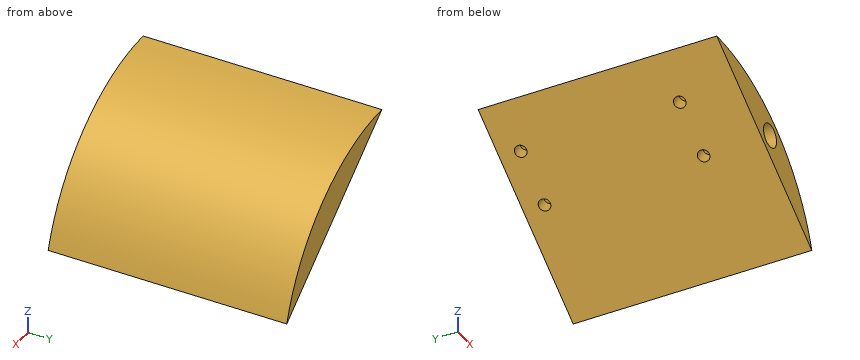
from build123d import *

# Parameters (mm, degrees)
SKETCH1_R           = 85.725
BOSS_EXTRUDE1_DEPTH = 114.3
CUT_EXTRUDE1_DEPTH  = 152.4
SKETCH3_R           = 2.778125
CUT_EXTRUDE2_DEPTH  = 7.9375
SKETCH4_R           = 5.588
CUT_EXTRUDE3_DEPTH  = 6.096


with BuildPart() as part:
    # Sketch1 → Boss-Extrude1 (new body)
    with BuildSketch(Plane(origin=(0, 0, 0), x_dir=(1, 0, 0), z_dir=(0, 1, 0))):
        Circle(SKETCH1_R)
    extrude(amount=BOSS_EXTRUDE1_DEPTH)

    # Sketch2 → Cut-Extrude1 (cut)
    with BuildSketch(Plane(origin=(0, 114.3, 0), x_dir=(1, 0, 0), z_dir=(0, 1, 0))):
        Polygon((0, -85.725), (81.83903771, -25.517592593), (151.304734273, 75.062868172), (-38.51393236, 115.934796391), (-149.339737724, 18.86396687), (-68.774879215, -104.537816407), align=None)
    extrude(amount=-CUT_EXTRUDE1_DEPTH, mode=Mode.SUBTRACT)

    # Sketch3 → Cut-Extrude2 (cut)
    with BuildSketch(Plane(origin=(40.919518855, 0, 55.621296296), x_dir=(-0.80550234, 0, 0.592592593), z_dir=(-0.592592593, 0, -0.80550234))):
        with Locations((2.54, 104.14)):
            Circle(SKETCH3_R)
        with Locations((27.94, 104.14)):
            Circle(SKETCH3_R)
        with Locations((2.54, 27.94)):
            Circle(SKETCH3_R)
        with Locations((27.94, 27.94)):
            Circle(SKETCH3_R)
    extrude(amount=-CUT_EXTRUDE2_DEPTH, mode=Mode.SUBTRACT)

    # Sketch4 → Cut-Extrude3 (cut)
    with BuildSketch(Plane(origin=(0, 0, 0), x_dir=(-1, 0, 0), z_dir=(0, -1, 0))):
        with Locations((-45.859759427, -62.336492182)):
            Circle(SKETCH4_R)
    extrude(amount=-CUT_EXTRUDE3_DEPTH, mode=Mode.SUBTRACT)


solid = part.part
The listing builds one solid part. Answer for the finished solid, in the listing's coordinates (mm). Coordinates: 2 decimals unless noted, no trailing zeros. Write each loop counter-clockwise with the first axis right and the second up, starting at its lowest first coordinate (ties: lowest second). Pieces come first, ordered by that corner, then holes. Notation, with made-up numbers: (60.25, 83.25) - (108.25, 83.25) arc R28 cw to (108.25, 111.25) - close; hole circle Ø2 at (14.5, -14.75). An arc over 180 degrees is marked (long way). Return JSON: item names as keys, results as strings.
1. Consider line 1 along X through (y, z) = (24.5, 58.5); line 2 along Z through (x, y) = (70, 58); line 3 along X through (y, z) = (86, 47.5). Determine where each line is inside the solid, lowest interval first.
Final values:
{"line 1": "37.01 to 62.66", "line 2": "34.23 to 49.49", "line 3": "51.96 to 71.36"}
2. Each of these flat-tipped pins is pushed along its axis until it touches: pin 1 Ø1 at (y, z) = (11.5, 60) entering from +X; pin 2 Ø2 at (x, y) = (66, 47.5) entering from -Z; pin 3 Ø5.5 at (x, z) = (45.5, 63.5) entering from -Y. Where does it stop, or does it pass through?
Final values:
{"pin 1": "x = 61.71", "pin 2": "z = 36.43", "pin 3": "y = 6.1"}
3. The part is cut by section C-C on z = 53. Determine the outline of the cut face in (x, y).
Final values:
{"outline": "(44.48, 0) - (67.38, 0) - (67.38, 114.3) - (44.48, 114.3) - close"}
4. The part is cut by section A-A on y = 78. Determine the outline of the cut face in (x, z) (3 decimals), then the cut area to 3 significant figures.
Final values:
{"outline": "(0, 85.725) - (81.839, 25.518) arc R85.725 ccw to start", "area": "1,150 mm^2"}
5. The part is cut by section B-B on x = 31.5. Determine the outline of the cut face in (y, z).
Final values:
{"outline": "(0, 62.55) - (114.3, 62.55) - (114.3, 79.73) - (0, 79.73) - close"}
